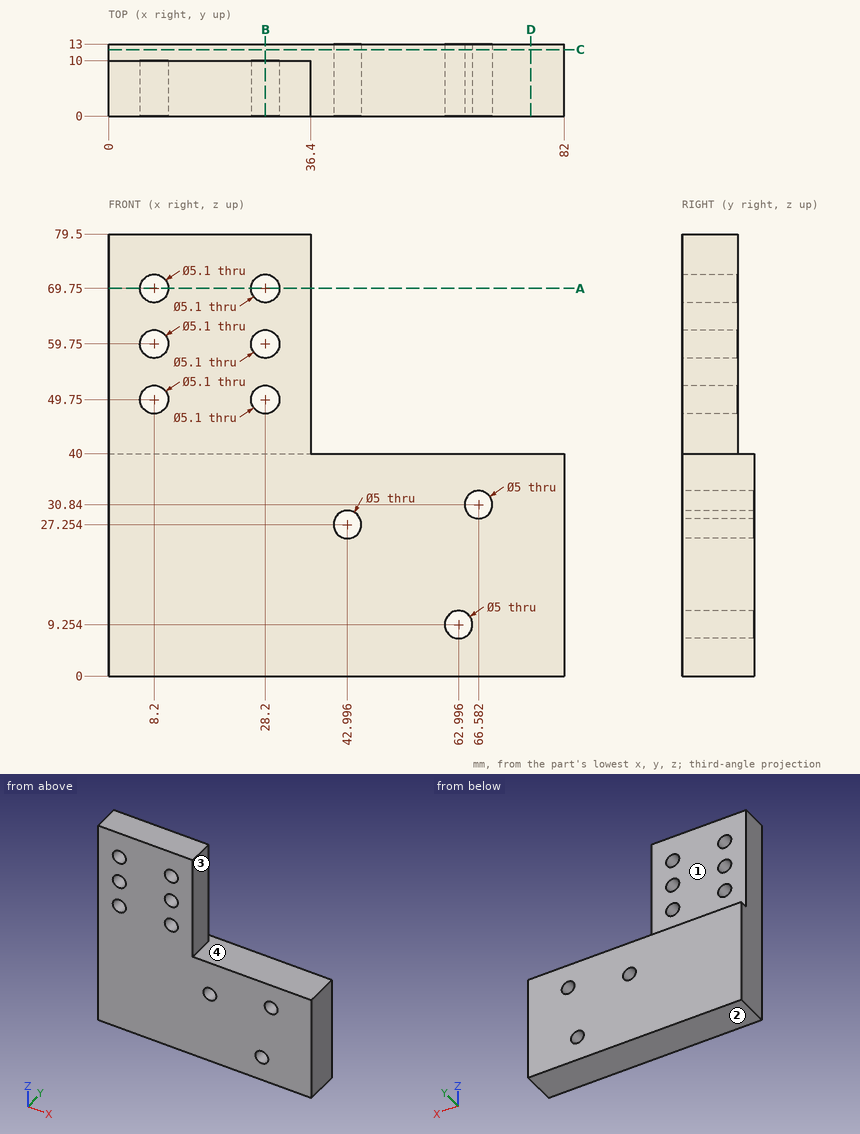
Can you work these out from the drawing? Everything is in mm from the part's minimum corner. A direction names the side the tool comes from. Give positions to 0.01 mm unless a question says otherwise; leave off trailing zeros. Write each loop counter-clockwise with the first axis right and the second up, starting at its lowest first coordinate (ties: lowest second). Pieces come first, ordered by that corner, then holes. Notation, with made-up numbers: M 86,-21.5 L 104,-21.5 A13 ccw 104,-13.5 Z; hole C 86.5,29 d11. An arc over 180 degrees is marked long. Answer in a Markdown table with one row per item. Add a question column.
Item 1: Imagine slicing it at D-D, the plane x = 76. Write out the boundary of the cut face in (y, z), plus the area to 3 significant figures.
Item 2: Please list where these lines run through material, in increasing order: L1, parallel to X at y = 5, z = 59.75; L2, parallel to Z at x = 38.5, y = 10.5; L3, parallel to X at y = 3, z = 71.5 (1 decimal).
Item 3: Imagine slicing it at A-A, the plane z = 69.75. Write out the boundary of the cut face in (x, y).
Item 4: Imagine slicing it at B-B, the plane x = 28.2. Write out the boundary of the cut face in (y, z), plus the area to 3 significant figures.
Item 5: For pin 1 Ø6 at (x, z) = (28.2, 59.75) entering from +Y; pin 2 Ø3 at (y, z) = (9.5, 58.5) entering from +X; pin 3 Ø3 at (x, y) = (65.5, 6.5) entering from +Z, each with a flat end and sliding along its axis, tell me the tip position at first contact or that it passes through.
Item 6: Imagine slicing it at C-C, the plane y = 12. Write out the boundary of the cut face in (x, z) (1 decimal), plus the area to 3 significant figures.
Item 7: On a 3-axis mill with a long thin cutter (end or side, diameter ignored), from which of +Z, -Z, +X, -X, +Y, -Y can I reach the whole of each face in a straight line? I mean the marked faces 1, 2, 3 and 4. Say none if no direction works.
Evaluation:
| question | item | result |
|---|---|---|
| 1 | outline | M 0,0 L 13,0 L 13,40 L 0,40 Z |
| 1 | area | 520 mm² |
| 2 | L1 | x = 0 to 5.65, 10.75 to 25.65, 30.75 to 36.4 |
| 2 | L2 | z = 0 to 40 |
| 2 | L3 | x = 0 to 6.3, 10.1 to 26.3, 30.1 to 36.4 |
| 3 | outline | M 0,0 L 5.65,0 L 5.65,10 L 0,10 Z; M 10.75,0 L 25.65,0 L 25.65,10 L 10.75,10 Z; M 30.75,0 L 36.4,0 L 36.4,10 L 30.75,10 Z |
| 4 | outline | M 0,0 L 13,0 L 13,40 L 10,40 L 10,47.2 L 0,47.2 Z; M 0,52.3 L 10,52.3 L 10,57.2 L 0,57.2 Z; M 0,62.3 L 10,62.3 L 10,67.2 L 0,67.2 Z; M 0,72.3 L 10,72.3 L 10,79.5 L 0,79.5 Z |
| 4 | area | 762 mm² |
| 5 | pin 1 | stops at y = 10 |
| 5 | pin 2 | stops at x = 36.4 |
| 5 | pin 3 | stops at z = 40 |
| 6 | outline | M 0,0 L 82,0 L 82,40 L 0,40 Z; hole C 43,27.3 d5; hole C 63,9.3 d5; hole C 66.6,30.8 d5 |
| 6 | area | 3,220 mm² |
| 7 | face 1 | +Z, +X, -X, +Y |
| 7 | face 2 | -Z, +X, -X, +Y, -Y |
| 7 | face 3 | +Z, +X, +Y, -Y |
| 7 | face 4 | +Z, +X, +Y |
